Could you check a few things on this model? Use its own coordinates, in mm. A direction names the side the tool comes from. Give positions to 0.01 mm unless a question says otherwise; leave off trailing zeros. Loops run counter-clockwise (first coordinate to the right, second up) from the corner with the lowest first, then second, coordinate; pieces in that order, holes last. Notation, with made-up numbers: (8, 42.5) -> (14, 42.5) arc R19 ccw to (14, 58.5) -> close; hole circle Ø10 at (63, -29.75). An arc over 180 degrees is marked (long way). Write each question's results on one line, items separated by ' | '. Start each with the question number.
Q1. If we section it at D-D, the plane x = 1.35: List the corners of the cut face in (y, z) for me, plus the area to 3 significant figures.
Q2. We'd pull the mould along X, two halves only. Please class faces 5 (the face through (0, 5, 2)), 6 (the face through (0.75, -5, -1)), 7 (the face through (0, 5, -2)), 8 (the face through (-1, 15, -1)): released by +X, released by -X, zero draft, split by the parting line, or undercut.
Q3. If I drill on line 1 along X through (y, z) = (5.25, -0.15) (3 decimals); line 2 along X through (y, z) = (-1.75, -0.85); line 3 along Y through (x, z) = (1.35, -1), over which ranges is the centre line in solid material (lowest first)?
Q4. Will these pins go through, and if not, where does the flat tip stop? P1, Ø0.8, axis at x = 0, z = -0.5, coming from the +Y side; P2, Ø0.8, axis at x = -1.5, y = 13, coming from the -Z side; P3, Ø0.5, axis at x = 1.5, y = 13, coming from the -Z side.
Q5. If we section it at B-B, the plane z = 0: List the corners of the cut face in (x, y) for me.
Q6. If we section it at A-A, the plane y = 13.25: List the corners of the cut face in (x, z) for me.
Q7. Which directions (+Z, -Z, +X, -X, +Y, -Y) give clear straight access to the entire face, cutting with the end or side of a thin tool? Please do faces 1 (the face through (0.02, -4.54, 2.75)), 2 (the face through (-1, -5, -0.75)), 3 (the face through (-1, 13, -0.5)), 4 (the face through (0.01, 2.79, 1.75)).
Q8. If we section it at C-C, the plane y = 3.5: List the corners of the cut face in (x, z) for me.
from build123d import *

# Parameters (mm, degrees)
SKETCH1_R           = 2.25
BOSS_EXTRUDE1_DEPTH = 15
SKETCH2_R           = 2.8
BOSS_EXTRUDE2_DEPTH = 0.6
CUT_EXTRUDE1_DEPTH  = 6.05
CUT_EXTRUDE5_DEPTH  = 6.05
CUT_EXTRUDE6_DEPTH  = 100
SKETCH11_W          = 1.5
SKETCH11_H          = 1.5
BOSS_EXTRUDE3_DEPTH = 8


with BuildPart() as part:
    # Sketch1 → Boss-Extrude1 (new body)
    with BuildSketch(Plane(origin=(0, 0, 0), x_dir=(1, 0, 0), z_dir=(0, 1, 0))):
        Circle(SKETCH1_R)
    extrude(amount=BOSS_EXTRUDE1_DEPTH)

    # Sketch2 → Boss-Extrude2 (add)
    with BuildSketch(Plane.XZ):
        Circle(SKETCH2_R)
    extrude(amount=BOSS_EXTRUDE2_DEPTH)

    # Sketch3 → Cut-Extrude1 (cut, through all)
    with BuildSketch(Plane.ZY.offset(2.25)):
        with BuildLine():
            Line((-0.5, 12), (-0.5, 15))
            ThreePointArc((-0.5, 15), (0, 15.5), (0.5, 15))
            Line((0.5, 15), (0.5, 12))
            ThreePointArc((0.5, 12), (0, 11.5), (-0.5, 12))
        make_face()
    extrude(amount=-CUT_EXTRUDE1_DEPTH, mode=Mode.SUBTRACT)

    # Sketch6 → Cut-Extrude5 (cut, through all)
    with BuildSketch(Plane.XY.offset(2.25)):
        with BuildLine():
            Line((-0.5, 5.5), (-0.5, 10.9))
            ThreePointArc((-0.5, 10.9), (0, 11.4), (0.5, 10.9))
            Line((0.5, 10.9), (0.5, 5.5))
            ThreePointArc((0.5, 5.5), (0, 5), (-0.5, 5.5))
        make_face()
    extrude(amount=-CUT_EXTRUDE5_DEPTH, mode=Mode.SUBTRACT)

    # Sketch8 → Cut-Extrude6 (cut)
    with BuildSketch(Plane(origin=(0, 100, 0), x_dir=(1, 0, 0), z_dir=(0, 1, 0))):
        with BuildLine():
            Line((0.5, 1.25), (0.5, -1.25))
            ThreePointArc((0.5, -1.25), (0, -1.75), (-0.5, -1.25))
            Line((-0.5, -1.25), (-0.5, 1.25))
            ThreePointArc((-0.5, 1.25), (0, 1.75), (0.5, 1.25))
        make_face()
    extrude(amount=-CUT_EXTRUDE6_DEPTH, mode=Mode.SUBTRACT)

    # Sketch11 → Boss-Extrude3 (add)
    with BuildSketch(Plane.XZ.offset(0.6)):
        with BuildLine():
            Line((-0.75, 2), (-0.75, 0.75))
            Line((-0.75, 0.75), (0.75, 0.75))
            Line((0.75, 0.75), (0.75, 2))
            ThreePointArc((0.75, 2), (0, 2.75), (-0.75, 2))
        make_face()
        Rectangle(SKETCH11_W, SKETCH11_H)
        with BuildLine():
            Line((0.75, 0.75), (0.75, -0.75))
            Line((0.75, -0.75), (2, -0.75))
            ThreePointArc((2, -0.75), (2.75, 0), (2, 0.75))
            Line((2, 0.75), (0.75, 0.75))
        make_face()
        with BuildLine():
            Line((-2, -0.75), (-0.75, -0.75))
            Line((-0.75, -0.75), (-0.75, 0.75))
            Line((-0.75, 0.75), (-2, 0.75))
            ThreePointArc((-2, 0.75), (-2.75, 0), (-2, -0.75))
        make_face()
        with BuildLine():
            Line((-0.75, -0.75), (-0.75, -2))
            ThreePointArc((-0.75, -2), (0, -2.75), (0.75, -2))
            Line((0.75, -2), (0.75, -0.75))
            Line((0.75, -0.75), (-0.75, -0.75))
        make_face()
    extrude(amount=BOSS_EXTRUDE3_DEPTH)


solid = part.part
Final values:
1) outline: (-8.6, -0.75) -> (-0.6, -0.75) -> (-0.6, -2.45) -> (0, -2.45) -> (0, -1.8) -> (15, -1.8) -> (15, -0.5) -> (12, -0.5) arc R0.5 cw to (12, 0.5) -> (15, 0.5) -> (15, 1.8) -> (0, 1.8) -> (0, 2.45) -> (-0.6, 2.45) -> (-0.6, 0.75) -> (-8.6, 0.75) -> close | area: 65.6 mm²
2) face 5: undercut | face 6: released by +X | face 7: undercut | face 8: zero draft
3) line 1: x = -2.245 to -0.5, 0.5 to 2.245 | line 2: x = -0.75 to 0.75 | line 3: y = -0.6 to 15
4) P1: stops at y = 0 | P2: stops at z = -1.96 | P3: stops at z = -1.87
5) outline: (-2.8, -0.6) -> (-2.75, -0.6) -> (-2.75, -8.6) -> (2.75, -8.6) -> (2.75, -0.6) -> (2.8, -0.6) -> (2.8, 0) -> (2.25, 0) -> (2.25, 11.5) -> (0.5, 11.5) -> (0.5, 0) -> (-0.5, 0) -> (-0.5, 11.5) -> (-2.25, 11.5) -> (-2.25, 0) -> (-2.8, 0) -> close
6) outline: (-2.19, -0.5) arc R2.25 ccw to (2.19, -0.5) -> (0.5, -0.5) -> (0.5, -1.25) arc R0.5 cw to (-0.5, -1.25) -> (-0.5, -0.5) -> close; (-2.19, 0.5) -> (-0.5, 0.5) -> (-0.5, 1.25) arc R0.5 cw to (0.5, 1.25) -> (0.5, 0.5) -> (2.19, 0.5) arc R2.25 ccw to start
7) face 1: +Z, -Y | face 2: -Z, -X, -Y | face 3: +X, -X, +Y | face 4: +Y
8) outline: circle Ø4.5 at (0, 0); hole (-0.5, -1.25) arc R0.5 ccw to (0.5, -1.25) -> (0.5, 1.25) arc R0.5 ccw to (-0.5, 1.25) -> close
